Autodesk Inventor part; units mm, degrees
ref_plane "Work Plane1" through (0, 0, -15) normal (0, 0, 1) x (1, 0, 0)
ref_plane "YZ Plane" through (0, 0, 0) normal (1, 0, 0) x (0, 1, 0)
ref_plane "XZ Plane" through (0, 0, 0) normal (0, 1, 0) x (-1, 0, 0)
sketch "Sketch1" plane through (0, 0, 0) normal (0, 0, 1) x (1, 0, 0)
  line L0 (0, 0) -> (25, 0)
  line L1 (25, 0) -> (25, 40)
  line L2 (25, 40) -> (0, 40)
  line L3 (0, 40) -> (0, 0)
  dimension "d1" = 25
  dimension "d2" = 40
  dimension "d3" = 25
extrude "Extrusion1" add sketch "Sketch1" against normal blind 30
sketch "Sketch2" plane through (25, 0, 0) normal (1, 0, 0) x (0, 0, -1)
  line L0 (0, 0) -> (30, 0)
  circle A0 centre (15, 6.56) radius 2.46
extrude "Extrusion2" cut sketch "Sketch2" against normal blind 30
sketch "Sketch3" plane through (0, 0, 0) normal (-1, 0, 0) x (0, 0, 1)
  line L0 (0, 0) -> (-30, 0)
  line L1 (-25.05, 0) -> (-4.95, 0)
  line L2 (-4.95, 0) -> (-4.95, 33.12)
  line L3 (-4.95, 33.12) -> (-25.05, 33.12)
  line L4 (-25.05, 33.12) -> (-25.05, 0)
  dimension "d11" = 20.1
extrude "Extrusion3" cut sketch "Sketch3" against normal blind 20
sketch "Sketch4" plane through (0, 0, 0) normal (0, -1, 0) x (1, 0, 0)
  line L0 (20, -4.95) -> (20, -25.05)
  line L1 (20, -15) -> (25, -15)
  line L2 (25, 0) -> (25, -30)
  line L3 (20, -8.025) -> (25, -8.025)
  line L4 (25, -8.025) -> (25, -21.975)
  line L5 (25, -21.975) -> (20, -21.975)
  line L6 (20, -21.975) -> (20, -8.025)
  line L7 (20, -8.025) -> (25, -21.975) construction
  line L8 (25, -8.025) -> (20, -21.975) construction
  line L9 (25, -12.54) -> (25, -17.46)
  point P0 (0, 0)
  point P1 (22.5, -15)
  dimension "d14" = 13.95
extrude "Extrusion4" add sketch "Sketch4" along normal blind 15
sketch "Sketch5" plane through (20, 0, 0) normal (-1, 0, 0) x (0, 0, 1)
  circle A0 centre (-15, 6.56) radius 2.46
  circle A1 centre (-15, 6.56) radius 4.7025
  circle A2 centre (-15, 6.56) radius 2.46
  circle A3 centre (-15, 6.56) radius 2.46
  point P0 (0, 0)
  dimension "d17" = 9.405
extrude "Extrusion5" cut sketch "Sketch5" against normal blind 2.1
sketch "Sketch6" plane through (25, 0, 0) normal (1, 0, 0) x (0, 0, -1)
  circle A0 centre (15, 6.56) radius 4.7025
  line L0 (15, 6.56) -> (15, 23.56)
  circle A1 centre (15, 23.56) radius 2.46
  point P0 (0, 0)
  dimension "d20" = 17
  dimension "d21" = 4.92
extrude "Extrusion6" cut sketch "Sketch6" against normal blind 10 contours A1
sketch "Sketch7" plane through (20, 0, 0) normal (-1, 0, 0) x (0, 0, 1)
  circle A0 centre (-15, 23.56) radius 2.46
  circle A1 centre (-15, 23.56) radius 4.7025
  point P0 (0, 0)
  dimension "d24" = 9.405
extrude "Extrusion7" cut sketch "Sketch7" against normal blind 2.1
sketch "Sketch9" plane through (25, 0, 0) normal (1, 0, 0) x (0, 0, -1)
  circle A0 centre (15, 6.56) radius 2.46
  circle A1 centre (15, 6.56) radius 2.46
  circle A2 centre (15, 23.56) radius 2.46
  circle A3 centre (15, 23.56) radius 2.46
  line L0 (30, 40) -> (30, 0)
  line L1 (30, 0) -> (30, 40)
  line L2 (30, 40) -> (0, 40)
  line L3 (0, 40) -> (0, 0)
  line L4 (0, 0) -> (8.025, 0)
  line L5 (21.975, 0) -> (21.975, -15)
  line L6 (21.975, -15) -> (8.025, -15)
  line L7 (8.025, -15) -> (8.025, 0)
  line L8 (0, 0) -> (8.025, 0)
  line L9 (21.975, 0) -> (30, 0)
extrude "Extrusion8" add sketch "Sketch9" along normal blind 5
sketch "Sketch10" plane through (0, 40, 0) normal (0, 1, 0) x (1, 0, 0)
  line L0 (0, 30) -> (30, 30)
  line L1 (30, 0) -> (0, 0)
  line L2 (0, 30) -> (30, 30)
  line L3 (30, 30) -> (30, 0)
  line L4 (30, 0) -> (0, 0)
  line L5 (0, 0) -> (0, 30)
extrude "Extrusion9" add sketch "Sketch10" along normal blind 30
sketch "Sketch12" plane through (30, 0, 0) normal (1, 0, 0) x (0, 0, -1)
  circle A0 centre (15, 6.56) radius 2.46
  line L0 (15, 6.56) -> (15, 15.06)
  circle A1 centre (15, 15.06) radius 2.525
  point P0 (0, 0)
  dimension "d31" = 8.5
  dimension "d33" = 5.05
extrude "Extrusion10" cut sketch "Sketch12" against normal blind 30 contours A1
sketch "Sketch14" plane through (0, 0, 0) normal (0, 0, 1) x (1, 0, 0)
  line L0 (30, 70) -> (0, 70)
  line L1 (0, 70) -> (0, 100)
  line L2 (30, 0) -> (30, 70)
  line L3 (30, 122.5) -> (30, 70)
  line L4 (30, 105) -> (30, 100)
  line L5 (-12, 145) -> (15, 145)
  line L6 (-7, 142.5) -> (-12, 145)
  line L7 (-7, 102.5) -> (-12, 100)
  line L8 (-7, 102.5) -> (-2, 122.5)
  line L9 (-2, 122.5) -> (-7, 142.5)
  line L10 (30, 122.5) -> (15, 145)
  line L11 (0, 100) -> (-12, 100)
  point P0 (0, 0)
  dimension "d86" = 12
extrude "Extrusion12" add sketch "Sketch14" against normal blind 30
sketch "Sketch15" plane through (0, 0, -25.05) normal (-1, 0, 0) x (0, 0, 1)
  line L0 (0, 33.12) -> (20.1, 33.12)
  line L1 (20.1, 33.12) -> (20.1, 0)
  line L2 (0, 33.12) -> (20.1, 33.12)
  line L3 (20.1, 33.12) -> (20.1, 31.1)
  line L4 (20.1, 31.1) -> (0, 31.1)
  line L5 (0, 31.1) -> (0, 33.12)
  point P0 (25.05, 0)
  dimension "d57" = 2.02
extrude "Extrusion13" add sketch "Sketch15" against normal blind 20
sketch "Sketch24" plane through (0, 0, 0) normal (0, 0, 1) x (1, 0, 0)
  line L0 (0, 100) -> (-12, 100)
  line L1 (-12, 100) -> (-7, 102.5)
  line L2 (0, 100) -> (-12, 100)
  line L3 (-12, 100) -> (-7, 102.5)
  line L4 (-7, 102.5) -> (-2, 122.5)
  line L5 (-7, 102.5) -> (-2, 122.5)
  line L6 (-2, 122.5) -> (-7, 142.5)
  line L7 (-2, 122.5) -> (-7, 142.5)
  line L8 (-7, 142.5) -> (-12, 145)
  line L9 (-7, 142.5) -> (-12, 145)
  line L10 (-12, 145) -> (15, 145)
  line L11 (-12, 145) -> (15, 145)
  line L12 (15, 145) -> (30, 122.5)
  line L13 (15, 145) -> (30, 122.5)
  line L14 (30, 122.5) -> (30, 87.5)
  line L15 (30, 87.5) -> (0, 87.5)
  line L16 (0, 87.5) -> (0, 100)
  point P0 (0, 0)
  dimension "d87" = 35
  dimension "d88" = 30
extrude "Extrusion14" add sketch "Sketch24" along normal blind 30
ref_plane "Work Plane1" through (0, 0, -15) normal (0, 0, 1) x (1, 0, 0)
mirror "Mirror1" about plane through (0, 0, -15) normal (0, 0, 1) of "Extrusion14"
properties part number "rec_b_40mm_x_90mm"
CAD build for the part. Positions are in the model's coordinates, mm. A direction names the side the tool comes from. Round coordinates to 2 decimals unless told otherwise and drop trailing zeros. Order: outer loops, then holes, each group sorted by start corner. A loop starts at its lowest first (then second) coordinate and runs counter-clockwise, first axis right, second up.
Q1. Slice it at B-B (y = 15.06). Write the cut outline in (x, z) (3 decimals), and give its area (4 significant figures).
Q2. Two-plate mould, pull along Y, no slides. Class faces 5 (the cylindrical face through (25.995, 7.502, -17.272)), 6 (the flat face through (10, 15, -4.95)), 7 (the flat face through (2, 145, -14)), 8 (the flat face through (15, 87.5, 15)): pulls with the +Y half, pulls with the -Y half, needs draft (parallel to the pull), parting line crosses it, or undercut.
Q3. Slice it at C-C (x = 24.5). Write the cut outline in (y, z) (3 decimals), and give its area (3 significant figures).
Q4. Slice it at A-A (z = -15). State how many separate pieces and enclosed holes the cut face has, and give its area (3 significant figures).
Q5. Slice it at D-D (z = 2.5). Write the cut outline in (x, y), and give its area (3 significant figures).
Q6. Which spindle directions (+Z, -Z, +X, -X, +Y, -Y) get a long thin tool onto all of the face, cutting with end or side? Do faces 1 (the flat face through (0, 65, -15)), 2 (the flat face through (10, 16, -25.05)), 3 (the flat face through (15, 44, -30)), 4 (the flat face through (15, 44, 0)). Say none if no direction does.
Q7. Wall check: L1, parallel to Z at x = 7.5, y = 8.5; L2, parallel to Y at x = 27, z = -15 (3 decimals); L3, parallel to Z at x = 21, y = 23. Give the ranges that are in metal, low to high.
Q8. Drop flat-ended pins along their axis: pin 1 (7.5 mm diameter, centred on y = 23.5, z = -13.5, fed in from -X); pin 2 (5 mm diameter, centred on x = 23.5, y = -9.5, fed in from -Z) (3 decimals); pin 3 (24 mm diameter, centred on x = 19, z = -44.5, fed in from -Y). Give the stop position or say it passes through.
Results below:
1. outline: (0, -30) - (30, -30) - (30, -17.525) - (20, -17.525) - (20, -25.05) - (0, -25.05) - close; (0, -4.95) - (20, -4.95) - (20, -12.475) - (30, -12.475) - (30, 0) - (0, 0) - close
1. area: 447.5 mm2
2. face 5: undercut
2. face 6: needs draft
2. face 7: pulls with the +Y half
2. face 8: pulls with the -Y half
3. outline: (-15, -21.975) - (0, -21.975) - (0, -30) - (87.5, -30) - (87.5, -60) - (130.75, -60) - (130.75, 30) - (87.5, 30) - (87.5, 0) - (0, 0) - (0, -8.025) - (-15, -8.025) - close; hole circle Ø4.92 at (6.56, -15); hole circle Ø5.05 at (15.06, -15); hole circle Ø4.92 at (23.56, -15)
3. area: 6,670 mm2
4. separate pieces: 4
4. enclosed holes: 0
4. area: 3,770 mm2
5. outline: (-12, 100) - (0, 100) - (0, 87.5) - (30, 87.5) - (30, 122.5) - (15, 145) - (-12, 145) - (-7, 142.5) - (-2, 122.5) - (-7, 102.5) - close
5. area: 1,780 mm2
6. face 1: +Z, -Z, -X, -Y
6. face 2: -X, -Y
6. face 3: -Z, +X, -X, -Y
6. face 4: +Z, +X, -X, -Y
7. L1: z = -30 to -25.05, -4.95 to 0
7. L2: y = -15 to 4.1, 9.02 to 12.535, 17.585 to 21.1, 26.02 to 127
7. L3: z = -30 to -19.67, -10.33 to 0
8. pin 1: stops at x = 20
8. pin 2: stops at z = -21.975
8. pin 3: stops at y = 87.5
